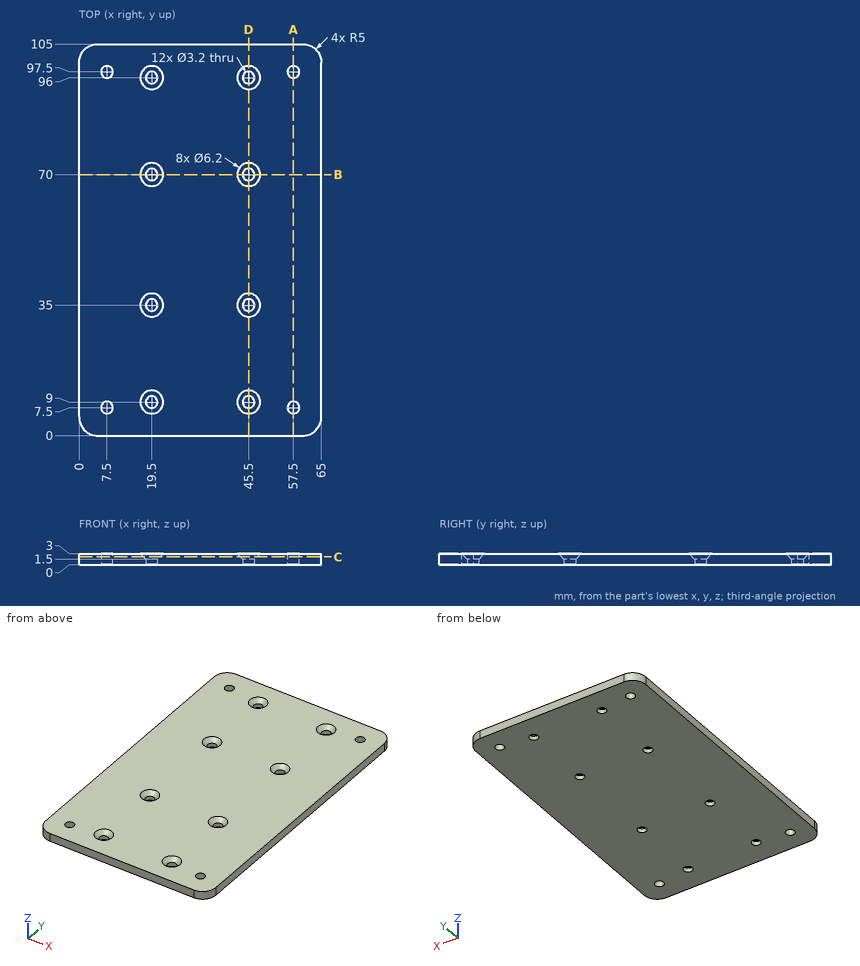
Design review of the part shown in the three views and the two pictorial views. Dimensions are in mm from the part's minimum x, y and z. Give positions to 0.01 mm unless a question says otherwise; leave off trailing zeros. Loops run counter-clockwise (first coordinate to the right, second up) from the corner with the lowest first, then second, coordinate; pieces in that order, holes last. Notation, with made-up numbers: (37, 34.5) - (52, 34.5) arc R12 ccw to (52, 39.5) - close; hole circle Ø8 at (71.5, 80.5). An arc over 180 degrees is marked (long way). Use CSV: the item, a comma, the result in double quotes. Start each with the question number.
1. Add section B-B (y = 70). State the section outline as (x, z) points, plus the area to 3 significant figures.
2. Add section A-A (x = 57.5). State the section outline as (y, z) points, plus the area to 3 significant figures.
3. Add section D-D (x = 45.5). State the section outline as (y, z) points, plus the area to 3 significant figures.
4. Wall thickness on L1, parallel to Y at x = 7.5, z = 1.75; L2, parallel to Y at x = 45.5, z = 0.75; L3, parallel to X at y = 34, z = 2.2: over which ranges is each line inside the solid? List them lowest first.
5. Add section C-C (z = 2.1). Count the separate pieces of the cut face and the enclosed holes in it, plus the area to 3 significant figures.
6. Insertion check: P1, Ø5, axis at x = 45.5, y = 9, coming from the -Z side. The pin has a flat end and moves straight along its axis. Give the tip position at first contact, or say it passes through.
Results found:
1,outline,"(0, 0) - (17.9, 0) - (17.9, 1.5) - (16.4, 3) - (0, 3) - close; (21.1, 0) - (43.9, 0) - (43.9, 1.5) - (42.4, 3) - (22.6, 3) - (21.1, 1.5) - close; (47.1, 0) - (65, 0) - (65, 3) - (48.6, 3) - (47.1, 1.5) - close"
1,area,"171 mm²"
2,outline,"(0, 0) - (5.9, 0) - (5.9, 3) - (0, 3) - close; (9.1, 0) - (95.9, 0) - (95.9, 3) - (9.1, 3) - close; (99.1, 0) - (105, 0) - (105, 3) - (99.1, 3) - close"
2,area,"296 mm²"
3,outline,"(0, 0) - (7.4, 0) - (7.4, 1.5) - (5.9, 3) - (0, 3) - close; (10.6, 0) - (33.4, 0) - (33.4, 1.5) - (31.9, 3) - (12.1, 3) - (10.6, 1.5) - close; (36.6, 0) - (68.4, 0) - (68.4, 1.5) - (66.9, 3) - (38.1, 3) - (36.6, 1.5) - close; (71.6, 0) - (94.4, 0) - (94.4, 1.5) - (92.9, 3) - (73.1, 3) - (71.6, 1.5) - close; (97.6, 0) - (105, 0) - (105, 3) - (99.1, 3) - (97.6, 1.5) - close"
3,area,"268 mm²"
4,L1,"y = 0 to 5.9, 9.1 to 95.9, 99.1 to 105"
4,L2,"y = 0 to 7.4, 10.6 to 33.4, 36.6 to 68.4, 71.6 to 94.4, 97.6 to 105"
4,L3,"x = 0 to 17.43, 21.57 to 43.43, 47.57 to 65"
5,separate pieces,"1"
5,enclosed holes,"12"
5,area,"6,650 mm²"
6,P1,"stops at z = 0"
